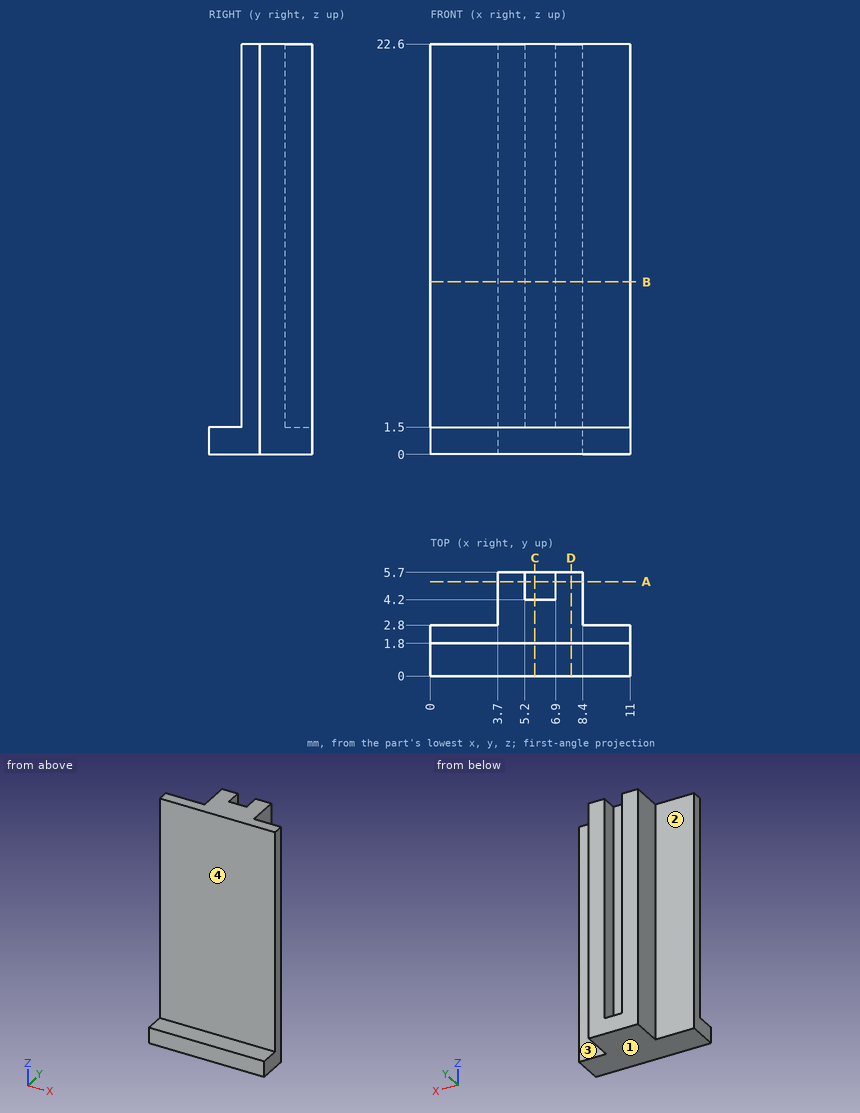
For this review, use the dimensioned drawing (mm, ordinates from the lowest corner) and the shaded views. A direction names the side the tool comes from. Give positions to 0.01 mm unless a question says otherwise; leave off trailing zeros. Order: outer loops, then holes, each group sorted by start corner. A loop starts at its lowest first (then second) coordinate and runs counter-clockwise, first axis right, second up. Notation, with made-up numbers: (57.5, -8.75) - (79.5, -8.75) arc R20 cw to (79.5, 29.25) - close; hole circle Ø3 at (-21, 19). An arc over 180 degrees is marked (long way). Use a Markdown table: item, result. Add a question column.
(1) Add section B-B on z = 9.5. Give the boundary of the cut face in (x, y), then the cut area to 3 significant figures.
(2) Machinability: for the marked faces 1, 2, 3 and 4, which of the approach directions +Z, -Z, +X, -X, +Y, -Y give a long, thin tool a straight path to every point of the face, cutting with its end or side? Answer none if there is none.
(3) Add section D-D on x = 7.75. Give the boundary of the cut face in (y, z).
(4) Wall thickness on probe 1 along X at (y, z) = (5.1, 14.25); probe 2 along Y at (x, z) = (10.5, 18.75); probe 3 along X at (y, z) = (3.6, 2): over which ranges is each line inside the solid? List them lowest first. Write a range as [from, to].
(5) Add section C-C on x = 5.75. Give the boundary of the cut face in (y, z), then the cut area to 3 significant figures.
(6) Clearance check with flat-ended pins moving along their axes: P1, Ø1.2, axis at y = 5, z = 12.5, coming from the -X side; P2, Ø0.9, axis at x = 7.5, y = 1, coming from the +Z side; P3, Ø1.4, axis at y = 4, z = 14, coming from the +X side. State where each tip first meets the part, or that it passes through.
(7) Add section A-A on y = 5.2. Give the boundary of the cut face in (x, z), then the cut area to 4 significant figures.
Report:
| question | item | result |
|---|---|---|
| 1 | outline | (0, 1.8) - (11, 1.8) - (11, 2.8) - (8.4, 2.8) - (8.4, 5.7) - (6.9, 5.7) - (6.9, 4.2) - (5.2, 4.2) - (5.2, 5.7) - (3.7, 5.7) - (3.7, 2.8) - (0, 2.8) - close |
| 1 | area | 22.1 mm² |
| 2 | face 1 | -Z, +X, -X, +Y, -Y |
| 2 | face 2 | +Z, -Z, -X, +Y |
| 2 | face 3 | +Z, -Z, +X, +Y |
| 2 | face 4 | +Z, +X, -X, -Y |
| 3 | outline | (0, 0) - (5.7, 0) - (5.7, 22.6) - (1.8, 22.6) - (1.8, 1.5) - (0, 1.5) - close |
| 4 | probe 1 | x = [3.7, 5.2], [6.9, 8.4] |
| 4 | probe 2 | y = [1.8, 2.8] |
| 4 | probe 3 | x = [3.7, 8.4] |
| 5 | outline | (0, 0) - (5.7, 0) - (5.7, 1.5) - (4.2, 1.5) - (4.2, 22.6) - (1.8, 22.6) - (1.8, 1.5) - (0, 1.5) - close |
| 5 | area | 59.2 mm² |
| 6 | P1 | stops at x = 3.7 |
| 6 | P2 | stops at z = 1.5 |
| 6 | P3 | stops at x = 8.4 |
| 7 | outline | (3.7, 0) - (8.4, 0) - (8.4, 22.6) - (6.9, 22.6) - (6.9, 1.5) - (5.2, 1.5) - (5.2, 22.6) - (3.7, 22.6) - close |
| 7 | area | 70.35 mm² |
